Geometry: final body of the model. Coordinates: model frame, mm. A direction names the side the tool comes from. Give positions to 0.01 mm unless a question says otherwise; leave off trailing zeros. Loops run counter-clockwise (first coordinate to the right, second up) from the corner with the lowest first, then second, coordinate; pieces in that order, holes last. Notation, with made-up numbers: (57, 89) - (67, 89) arc R18 ccw to (67, 118) - close; hole circle Ø2 at (18.25, 73.5). An arc over 180 degrees is marked (long way). Use one line per item in the form item = value.
```python
from build123d import *

# Parameters (mm, degrees)
BOSS_EXTRUDE1_DEPTH     = 3.175
FILLET1_R               = 50.8
SKETCH2_W               = 12.7
SKETCH2_H               = 3.175
CUT_EXTRUDE1_DEPTH      = 3.175
MIRROR2_COPY_1_SKETCH_W = 12.7
MIRROR2_COPY_1_SKETCH_H = 3.175
MIRROR2_COPY_1_DEPTH    = 3.175
CUT_EXTRUDE2_DEPTH      = 3.175
SKETCH4_W               = 63.5
SKETCH4_H               = 3.175
CUT_EXTRUDE3_DEPTH      = 3.175
MIRROR5_COPY_1_DEPTH    = 3.175
MIRROR5_COPY_2_DEPTH    = 3.175
SKETCH5_W               = 3.175
SKETCH5_H               = 12.7
CUT_EXTRUDE4_DEPTH      = 3.175
MIRROR7_COPY_1_SKETCH_W = 3.175
MIRROR7_COPY_1_SKETCH_H = 12.7
MIRROR7_COPY_1_DEPTH    = 3.175


with BuildPart() as part:
    # Sketch1 → Boss-Extrude1 (new body)
    with BuildSketch(Plane(origin=(0, 0, 0), x_dir=(1, 0, 0), z_dir=(0, 1, 0))):
        with BuildLine():
            ThreePointArc((-304.8, -228.6), (-289.921024484, -264.521024484), (-254, -279.4))
            Line((-254, -279.4), (-63.5, -279.4))
            ThreePointArc((-63.5, -279.4), (0, -215.9), (63.5, -279.4))
            Line((63.5, -279.4), (254, -279.4))
            ThreePointArc((254, -279.4), (289.921024484, -264.521024484), (304.8, -228.6))
            Line((304.8, -228.6), (304.8, -63.5))
            ThreePointArc((304.8, -63.5), (241.3, 0), (304.8, 63.5))
            Line((304.8, 63.5), (304.8, 228.6))
            ThreePointArc((304.8, 228.6), (289.921024484, 264.521024484), (254, 279.4))
            Line((254, 279.4), (63.5, 279.4))
            ThreePointArc((63.5, 279.4), (0, 215.9), (-63.5, 279.4))
            Line((-63.5, 279.4), (-254, 279.4))
            ThreePointArc((-254, 279.4), (-289.921024484, 264.521024484), (-304.8, 228.6))
            Line((-304.8, 228.6), (-304.8, 63.5))
            ThreePointArc((-304.8, 63.5), (-241.3, 0), (-304.8, -63.5))
            Line((-304.8, -63.5), (-304.8, -228.6))
        make_face()
    extrude(amount=BOSS_EXTRUDE1_DEPTH)

    # Fillet1
    fillet1_edges = [part.edges().sort_by_distance(p)[0] for p in [
        (-63.5, 1.5875, -279.4),
        (63.5, 1.5875, -279.4),
        (304.8, 1.5875, -63.5),
        (304.8, 1.5875, 63.5),
        (63.5, 1.5875, 279.4),
        (-63.5, 1.5875, 279.4),
        (-304.8, 1.5875, 63.5),
        (-304.8, 1.5875, -63.5),
    ]]
    fillet(fillet1_edges, radius=FILLET1_R)

    # Sketch2 → Cut-Extrude1 (cut)
    with BuildSketch(Plane(origin=(0, 3.175, 0), x_dir=(1, 0, 0), z_dir=(0, 1, 0))):
        with Locations((-171.45, 195.2625)):
            Rectangle(SKETCH2_W, SKETCH2_H)
        with Locations((-196.85, 195.2625)):
            Rectangle(SKETCH2_W, SKETCH2_H)
        with Locations((-146.05, 195.2625)):
            Rectangle(SKETCH2_W, SKETCH2_H)
    cut_extrude1 = extrude(amount=-CUT_EXTRUDE1_DEPTH, mode=Mode.SUBTRACT)

    # Mirror1: Cut-Extrude1 across plane
    add(cut_extrude1.mirror(Plane.XY), mode=Mode.SUBTRACT)

    # Mirror2: Cut-Extrude1 across plane
    add(cut_extrude1.mirror(Plane(origin=(0, 0, 0), x_dir=(0, 0, 1), z_dir=(1, 0, 0))), mode=Mode.SUBTRACT)

    # Mirror2 copy 1 sketch → Mirror2 copy 1 (cut)
    with BuildSketch(Plane(origin=(0, 3.175, 0), x_dir=(-1, 0, 0), z_dir=(0, 1, 0))):
        with Locations((-171.45, 195.2625)):
            Rectangle(MIRROR2_COPY_1_SKETCH_W, MIRROR2_COPY_1_SKETCH_H)
        with Locations((-196.85, 195.2625)):
            Rectangle(MIRROR2_COPY_1_SKETCH_W, MIRROR2_COPY_1_SKETCH_H)
        with Locations((-146.05, 195.2625)):
            Rectangle(MIRROR2_COPY_1_SKETCH_W, MIRROR2_COPY_1_SKETCH_H)
    extrude(amount=-MIRROR2_COPY_1_DEPTH, mode=Mode.SUBTRACT)

    # Sketch3 → Cut-Extrude2 (cut)
    with BuildSketch(Plane(origin=(0, 3.175, 0), x_dir=(1, 0, 0), z_dir=(0, 1, 0))):
        Polygon((-251.369743879, 152.653015062), (-260.35, 143.672758941), (-258.10493597, 141.42769491), (-249.124679849, 150.407951031), align=None)
        Polygon((-233.409231637, 170.613527304), (-242.389487758, 161.633271183), (-240.144423728, 159.388207153), (-231.164167607, 168.368463274), align=None)
        Polygon((-213.203655364, 186.328975516), (-222.183911485, 177.348719395), (-224.428975516, 179.593783425), (-215.448719395, 188.574039546), align=None)
    cut_extrude2 = extrude(amount=-CUT_EXTRUDE2_DEPTH, mode=Mode.SUBTRACT)

    # Sketch4 → Cut-Extrude3 (cut)
    with BuildSketch(Plane(origin=(0, 3.175, 0), x_dir=(1, 0, 0), z_dir=(0, 1, 0))):
        with Locations((0, 195.2625)):
            Rectangle(SKETCH4_W, SKETCH4_H)
        with Locations((0, -195.2625)):
            Rectangle(SKETCH4_W, SKETCH4_H)
    cut_extrude3 = extrude(amount=-CUT_EXTRUDE3_DEPTH, mode=Mode.SUBTRACT)

    # Mirror4: Cut-Extrude2 across plane
    add(cut_extrude2.mirror(Plane.XY), mode=Mode.SUBTRACT)

    # Mirror5: Cut-Extrude3 across plane
    add(cut_extrude3.mirror(Plane(origin=(0, 0, 0), x_dir=(0, 0, 1), z_dir=(1, 0, 0))), mode=Mode.SUBTRACT)

    # Mirror5 copy 1 sketch → Mirror5 copy 1 (cut)
    with BuildSketch(Plane(origin=(0, 3.175, 0), x_dir=(-1, 0, 0), z_dir=(0, 1, 0))):
        Polygon((-251.369743879, 152.653015062), (-260.35, 143.672758941), (-258.10493597, 141.42769491), (-249.124679849, 150.407951031), align=None)
        Polygon((-233.409231637, 170.613527304), (-242.389487758, 161.633271183), (-240.144423728, 159.388207153), (-231.164167607, 168.368463274), align=None)
        Polygon((-213.203655364, 186.328975516), (-222.183911485, 177.348719395), (-224.428975516, 179.593783425), (-215.448719395, 188.574039546), align=None)
    extrude(amount=-MIRROR5_COPY_1_DEPTH, mode=Mode.SUBTRACT)

    # Mirror5 copy 2 sketch → Mirror5 copy 2 (cut)
    with BuildSketch(Plane(origin=(0, 3.175, 0), x_dir=(-1, 0, 0), z_dir=(0, 1, 0))):
        Polygon((-251.369743879, -152.653015062), (-260.35, -143.672758941), (-258.10493597, -141.42769491), (-249.124679849, -150.407951031), align=None)
        Polygon((-233.409231637, -170.613527304), (-242.389487758, -161.633271183), (-240.144423728, -159.388207153), (-231.164167607, -168.368463274), align=None)
        Polygon((-213.203655364, -186.328975516), (-222.183911485, -177.348719395), (-224.428975516, -179.593783425), (-215.448719395, -188.574039546), align=None)
    extrude(amount=-MIRROR5_COPY_2_DEPTH, mode=Mode.SUBTRACT)

    # Sketch5 → Cut-Extrude4 (cut)
    with BuildSketch(Plane(origin=(0, 3.175, 0), x_dir=(1, 0, 0), z_dir=(0, 1, 0))):
        with Locations((-271.4625, -95.25)):
            Rectangle(SKETCH5_W, SKETCH5_H)
        with Locations((-271.4625, -69.85)):
            Rectangle(SKETCH5_W, SKETCH5_H)
        with Locations((-271.4625, -120.65)):
            Rectangle(SKETCH5_W, SKETCH5_H)
    cut_extrude4 = extrude(amount=-CUT_EXTRUDE4_DEPTH, mode=Mode.SUBTRACT)

    # Mirror6: Cut-Extrude4 across plane
    add(cut_extrude4.mirror(Plane(origin=(0, 0, 0), x_dir=(0, 0, 1), z_dir=(1, 0, 0))), mode=Mode.SUBTRACT)

    # Mirror7: Cut-Extrude4 across plane
    add(cut_extrude4.mirror(Plane.XY), mode=Mode.SUBTRACT)

    # Mirror7 copy 1 sketch → Mirror7 copy 1 (cut)
    with BuildSketch(Plane(origin=(0, 3.175, 0), x_dir=(-1, 0, 0), z_dir=(0, 1, 0))):
        with Locations((-271.4625, -95.25)):
            Rectangle(MIRROR7_COPY_1_SKETCH_W, MIRROR7_COPY_1_SKETCH_H)
        with Locations((-271.4625, -69.85)):
            Rectangle(MIRROR7_COPY_1_SKETCH_W, MIRROR7_COPY_1_SKETCH_H)
        with Locations((-271.4625, -120.65)):
            Rectangle(MIRROR7_COPY_1_SKETCH_W, MIRROR7_COPY_1_SKETCH_H)
    extrude(amount=-MIRROR7_COPY_1_DEPTH, mode=Mode.SUBTRACT)


solid = part.part
```
(1) Access query for faces 1 (the face through (297.378, 1.61, 75.953)), 2 (the face through (-75.953, 1.61, 271.978)), 3 (the face through (-297.378, 1.61, -75.953)), 4 (the face through (75.953, 1.61, -271.978)). Directions: +Z, -Z, +X, -X, +Y, -Y. A direction counts if a zero-diameter tool reaches every point of the face in a straight line with its end or side. Return the directions, or none.
Solution:
face_1 = +X, +Y, -Y
face_2 = +Z, +Y, -Y
face_3 = -X, +Y, -Y
face_4 = -Z, +Y, -Y
(2) Cut plane D-D (x = -64). Return the cut outline in (y, z) (3 decimals).
Solution:
outline = (0, -261.869) - (3.175, -261.869) - (3.175, 261.869) - (0, 261.869) - close
(3) Cut plane B-B (y = 1.3). Give the number of separate pieces and of enclosed holes in the cut face, plus the area to 3 significant figures.
Solution:
separate_pieces = 1
enclosed_holes = 38
area = 309,000 mm2
(4) Material intervals for L1, parallel to X at y = 2.95, z = -170.5; L2, parallel to Z at x = 214, y = 2.45; L3, parallel to Z at x = -10.5, y = 2 (3 decimals), sorted ascending. Write a range as from..to.
Solution:
L1 = -304.8..-233.52, -233.3..233.3, 233.52..304.8
L2 = -279.4..-187.13, -185.53..185.53, 187.13..279.4
L3 = -216.774..-196.85, -193.675..193.675, 196.85..216.774
(5) Cut plane C-C (z = -46.5). Return the cut outline in (x, y) (1 decimal), plus the area to 3 significant figures.
Solution:
outline = (-261.6, 0) - (261.6, 0) - (261.6, 3.2) - (-261.6, 3.2) - close
area = 1,660 mm2
(6) Pull-direction query (X, two-part tool) for faces 5 (the face through (-296.96, 1.61, 75.28)), 6 (the face through (289.524, 1.565, 264.914)), 7 (the face through (75.28, 1.61, 271.56)); classes: released by +X, released by -X, zero draft, split by the parting line, or undercut.
Solution:
face_5 = released by -X
face_6 = released by +X
face_7 = undercut
(7) Cut plane A-A (x = 20). Return the cut outline in (y, z) (3 decimals).
Solution:
outline = (0, -219.132) - (3.175, -219.132) - (3.175, -196.85) - (0, -196.85) - close; (0, -193.675) - (3.175, -193.675) - (3.175, 193.675) - (0, 193.675) - close; (0, 196.85) - (3.175, 196.85) - (3.175, 219.132) - (0, 219.132) - close
